Geometry check sheet. Reference: the model listing, model coordinates, mm. Face numbers are marked on the shaded views. A direction names the side the tool comes from. Round coordinates to 2 decimals unless told otherwise and drop trailing zeros. Write each loop counter-clockwise with the first axis right and the second up, starting at its lowest first coordinate (ties: lowest second). Pieces come first, ordered by that corner, then holes. Notation, with made-up numbers: (-14.5, 16) -> (44.5, 16) arc R6 cw to (44.5, 22) -> close; hole circle Ø8 at (77.5, -8). An arc over 180 degrees is marked (long way). Return JSON: item names as keys, results as strings. Group by question number.
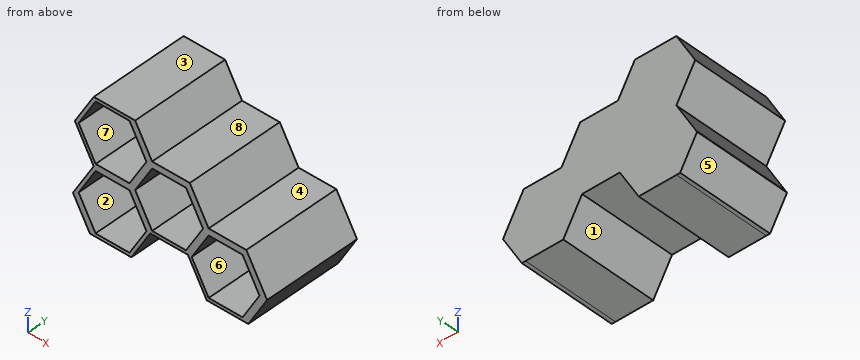
from build123d import *

# Parameters (mm, degrees)
F1_DEPTH = 12.7
F2_DEPTH = 95.25


# Not quite as in the source:
# - a feature names something its author has since deleted; it is built from what else it names


with BuildPart() as f1:
    # F0 (on Front) → F1 (new body)
    with BuildSketch(Plane.XZ):
        Polygon((87.3760877519, 66.7924993012), (50.7143456583, 66.7924993012), (32.3834746116, 35.0424993012), (50.7143456583, 3.2924993012), (87.3760877518, 3.2924993011), (105.7069587986, 35.0424993011), align=None)
        Polygon((52.547432763, 6.4674993012), (36.0496488209, 35.0424993012), (52.547432763, 63.6174993012), (85.5430006472, 63.6174993011), (102.0407845893, 35.0424993011), (85.5430006472, 6.4674993011), align=None, mode=Mode.SUBTRACT)
        Polygon((50.7143456583, 130.2924993012), (32.3834746116, 98.5424993012), (50.7143456583, 66.7924993012), (87.3760877519, 66.7924993012), (105.7069587986, 98.5424993012), (87.3760877519, 130.2924993012), align=None)
        Polygon((52.547432763, 69.9674993012), (36.0496488209, 98.5424993012), (52.547432763, 127.1174993012), (85.5430006472, 127.1174993012), (102.0407845893, 98.5424993012), (85.5430006472, 69.9674993012), align=None, mode=Mode.SUBTRACT)
        Polygon((160.699571939, 66.7924993012), (142.3687008922, 35.0424993012), (160.6995719389, 3.2924993011), (197.3613140325, 3.2924993011), (215.6921850793, 35.0424993012), (197.3613140325, 66.7924993012), align=None)
        Polygon((162.5326590436, 6.4674993012), (146.0348751015, 35.0424993012), (162.5326590436, 63.6174993012), (195.5282269278, 63.6174993012), (212.0260108699, 35.0424993012), (195.5282269278, 6.4674993012), align=None, mode=Mode.SUBTRACT)
        Polygon((105.7069587986, 98.5424993012), (87.3760877519, 66.7924993012), (105.7069587986, 35.0424993011), (142.3687008922, 35.0424993011), (160.699571939, 66.7924993012), (142.3687008922, 98.5424993012), align=None)
        Polygon((107.5400459033, 38.2174993012), (91.0422619612, 66.7924993012), (107.5400459033, 95.3674993012), (140.5356137875, 95.3674993012), (157.0333977296, 66.7924993012), (140.5356137875, 38.2174993012), align=None, mode=Mode.SUBTRACT)
        Polygon((52.547432763, 127.1174993012), (36.0496488209, 98.5424993012), (52.547432763, 69.9674993012), (85.5430006472, 69.9674993012), (102.0407845893, 98.5424993012), (85.5430006472, 127.1174993012), align=None)
        Polygon((52.547432763, 63.6174993012), (36.0496488209, 35.0424993012), (52.547432763, 6.4674993012), (85.5430006472, 6.4674993011), (102.0407845893, 35.0424993011), (85.5430006472, 63.6174993011), align=None)
        Polygon((162.5326590436, 63.6174993012), (146.0348751015, 35.0424993012), (162.5326590436, 6.4674993012), (195.5282269278, 6.4674993012), (212.0260108699, 35.0424993012), (195.5282269278, 63.6174993012), align=None)
        Polygon((107.5400459033, 95.3674993012), (91.0422619612, 66.7924993012), (107.5400459033, 38.2174993012), (140.5356137875, 38.2174993012), (157.0333977296, 66.7924993012), (140.5356137875, 95.3674993012), align=None)
    extrude(amount=F1_DEPTH)

    # F0 (on Front) → F2 (join)
    with BuildSketch(Plane.XZ):
        Polygon((50.7143456583, 130.2924993012), (32.3834746116, 98.5424993012), (50.7143456583, 66.7924993012), (87.3760877519, 66.7924993012), (105.7069587986, 98.5424993012), (87.3760877519, 130.2924993012), align=None)
        Polygon((52.547432763, 69.9674993012), (36.0496488209, 98.5424993012), (52.547432763, 127.1174993012), (85.5430006472, 127.1174993012), (102.0407845893, 98.5424993012), (85.5430006472, 69.9674993012), align=None, mode=Mode.SUBTRACT)
        Polygon((87.3760877519, 66.7924993012), (50.7143456583, 66.7924993012), (32.3834746116, 35.0424993012), (50.7143456583, 3.2924993012), (87.3760877518, 3.2924993011), (105.7069587986, 35.0424993011), align=None)
        Polygon((52.547432763, 6.4674993012), (36.0496488209, 35.0424993012), (52.547432763, 63.6174993012), (85.5430006472, 63.6174993011), (102.0407845893, 35.0424993011), (85.5430006472, 6.4674993011), align=None, mode=Mode.SUBTRACT)
        Polygon((105.7069587986, 98.5424993012), (87.3760877519, 66.7924993012), (105.7069587986, 35.0424993011), (142.3687008922, 35.0424993011), (160.699571939, 66.7924993012), (142.3687008922, 98.5424993012), align=None)
        Polygon((107.5400459033, 38.2174993012), (91.0422619612, 66.7924993012), (107.5400459033, 95.3674993012), (140.5356137875, 95.3674993012), (157.0333977296, 66.7924993012), (140.5356137875, 38.2174993012), align=None, mode=Mode.SUBTRACT)
        Polygon((160.699571939, 66.7924993012), (142.3687008922, 35.0424993012), (160.6995719389, 3.2924993011), (197.3613140325, 3.2924993011), (215.6921850793, 35.0424993012), (197.3613140325, 66.7924993012), align=None)
        Polygon((162.5326590436, 6.4674993012), (146.0348751015, 35.0424993012), (162.5326590436, 63.6174993012), (195.5282269278, 63.6174993012), (212.0260108699, 35.0424993012), (195.5282269278, 6.4674993012), align=None, mode=Mode.SUBTRACT)
        Polygon((91.0422619612, 130.2924993012), (87.3760877519, 130.2924993012), (105.7069587986, 98.5424993012), (142.3687008922, 98.5424993012), (160.699571939, 66.7924993012), (197.3613140325, 66.7924993012), (215.6921850793, 35.0424993012), (197.3613140325, 3.2924993012), (201.0274882418, 3.2924993011), (219.3583592886, 35.0424993012), (199.1944011372, 69.9674993012), (162.5326590436, 69.9674993012), (144.2017879969, 101.7174993012), (107.5400459033, 101.7174993012), align=None)
        Polygon((50.7143456583, 3.2924993012), (32.3834746116, 35.0424993012), (30.5503875069, 31.8674993012), (47.048171449, 3.2924993012), align=None)
    extrude(amount=F2_DEPTH)


solid = f1.part
1) Sectioned sample at B-B on z = 82. Enter the section's corners in (x, y).
2) Sectioned sample at D-D on y = -29.5. State how many separate pieces and enclosed holes the cut face has, and give its area (3 significant figures).
3) Go/stop test with flat-tipped pins: P1, Ø18.5, axis at x = 117.5, y = -56, coming from the -Z side; P2, Ø11, axis at x = 177, y = -64.5, coming from the +Z side; P3, Ø10, axis at x = 123.5, z = 46.5, coming from the -Y side. Record where each tip stops, or that it passes through.
4) Material ranges on probe 1 along Z at (x, y) = (79.5, -49); probe 2 along Z at (x, y) = (123.5, -60.5); probe 3 along X at (y, z) = (-90, 80.5), recorded low to high. Write a range as [from, to].
5) Tool access check on the marked faces 1, 2, 3 and 4. Record the directions out of +Z, -Z, +X, -X, +Y, -Y that give a thin tool (end or side, any length) a straight path to the whole face; none if there is none.
6) Mould release check, pull along X, two halves, no side actions. Record for the marked faces 5, 6, 7 and 8: +X half, -X half, draft (parallel to the pull), parting line (faces both ways), or undercut.
7) Sectioned sample at A-A on x = 76.5. Enter the section's corners in (y, z), and give its area (3 significant figures).
8) Sectioned sample at C-C on y = -8. Enter the section's corners in (x, z).
Evaluation:
{
 "1": {"outline": "(41.93, -95.25) -> (45.6, -95.25) -> (45.6, -12.7) -> (92.49, -12.7) -> (92.49, -95.25) -> (99.82, -95.25) -> (99.82, -12.7) -> (148.25, -12.7) -> (148.25, -95.25) -> (155.59, -95.25) -> (155.59, 0) -> (41.93, 0) -> close"},
 "2": {"separate pieces": "1", "enclosed holes": "4", "area": "3,460 mm2"},
 "3": {"P1": "stops at z = 35.04", "P2": "stops at z = 69.97", "P3": "stops at y = -12.7"},
 "4": {"probe 1": "z = [3.29, 6.47], [63.62, 69.97], [127.12, 130.29]", "probe 2": "z = [35.04, 38.22], [95.37, 101.72]", "probe 3": "x = [42.8, 46.47], [91.62, 98.96], [149.12, 156.45]"},
 "5": {"face 1": "-Z, +Y, -Y", "face 2": "-Y", "face 3": "+Z, +X, -X, +Y, -Y", "face 4": "+Z, +X, +Y, -Y"},
 "6": {"face 5": "-X half", "face 6": "undercut", "face 7": "undercut", "face 8": "draft"},
 "7": {"outline": "(-95.25, 3.29) -> (0, 3.29) -> (0, 130.29) -> (-95.25, 130.29) -> (-95.25, 127.12) -> (-12.7, 127.12) -> (-12.7, 69.97) -> (-95.25, 69.97) -> (-95.25, 63.62) -> (-12.7, 63.62) -> (-12.7, 6.47) -> (-95.25, 6.47) -> close", "area": "2,660 mm2"},
 "8": {"outline": "(30.55, 31.87) -> (47.05, 3.29) -> (87.38, 3.29) -> (105.71, 35.04) -> (142.37, 35.04) -> (160.7, 3.29) -> (201.03, 3.29) -> (219.36, 35.04) -> (199.19, 69.97) -> (162.53, 69.97) -> (144.2, 101.72) -> (107.54, 101.72) -> (91.04, 130.29) -> (50.71, 130.29) -> (32.38, 98.54) -> (50.71, 66.79) -> close"}
}
